Autodesk Inventor part; units mm, degrees
ref_plane "YZ Plane" through (0, 0, 0) normal (1, 0, 0) x (0, 1, 0)
ref_plane "XZ Plane" through (0, 0, 0) normal (0, 1, 0) x (-1, 0, 0)
ref_plane "XY Plane" through (0, 0, 0) normal (0, 0, 1) x (1, 0, 0)
sketch "Esquisse1" plane through (0, 0, 0) normal (0, 1, 0) x (-1, 0, 0)
  line L0 (0, 0) -> (20, 0)
  line L1 (20, 0) -> (20, -86)
  line L2 (20, -86) -> (0, -86)
  line L3 (0, -86) -> (0, 0)
  dimension "d0" = 86
  dimension "d1" = 20
extrude "Extrusion1" add sketch "Esquisse1" along normal blind 3
sketch "Esquisse2" plane through (0, 3, 0) normal (0, 1, 0) x (1, 0, 0)
  line L0 (-20, 0) -> (0, 0)
  line L1 (0, 0) -> (0, 86)
  line L2 (10.8927, 42.5) -> (-28.8955, 42.5) construction
  point P0 (-3, 6)
  dimension "d12" = 3
  dimension "d37" = 42.5
  dimension "d39" = 36.5
hole "Perçage1" at (-3, 3, -6) direction (0, -1, 0) diameter 3.5 end through all
pattern_linear "Réseau rectangulaire1" count 2 spacing 14 along (-1, 0, 0) count 2 spacing 74 along (0, 0, -1) of "Perçage1"
sketch "Esquisse3" plane through (0, 3, 0) normal (0, 1, 0) x (1, 0, 0)
  line L0 (-15.25, 31) -> (-2.75, 31)
  line L1 (-2.75, 31) -> (-2.75, 55)
  line L2 (-2.75, 55) -> (-15.25, 55)
  line L3 (-15.25, 55) -> (-15.25, 31)
  line L4 (0, 86) -> (-20, 86)
  line L5 (-20, 86) -> (-20, 0)
  point P0 (0, 0)
  dimension "d19" = 24
  dimension "d20" = 12.5
  dimension "d21" = 31
  dimension "d22" = 4.75
extrude "Extrusion2" cut sketch "Esquisse3" against normal through all
sketch "Esquisse4" plane through (0, 3, 0) normal (0, 1, 0) x (1, 0, 0)
  line L0 (-2.75, 55) -> (-2.75, 31)
  line L1 (-2.75, 31) -> (-15.25, 31)
  point P0 (0, 0)
  point P1 (-9, 29.15)
  dimension "d32" = 6.25
  dimension "d33" = 1.85
hole "Perçage2" at (-9, 3, -29.15) direction (0, -1, 0) diameter 2 end through all
pattern_linear "Réseau rectangulaire2" count 2 spacing 27.7 along (0, 0, -1) of "Perçage2"
properties part number "support_servo_moteur"
Build history of the part. All positions in model axes, mm. A direction names the side the tool comes from. Round coordinates to 2 decimals unless told otherwise and drop trailing zeros. Write each loop counter-clockwise with the first axis right and the second up, starting at its lowest first coordinate (ties: lowest second). Pieces come first, ordered by that corner, then holes. Notation, with made-up numbers: M 60.25,61.5 L 79.25,61.5 A17 ccw 79.25,78.5 Z; hole C 58,27.25 d8. An arc over 180 degrees is marked long. Answer as a JSON object with one key per item and string values. Group by question number.
(1) Cut at C-C (y = 0.95). Give the cut face in (x, z).
(2) Which spindle directions (+Z, -Z, +X, -X, +Y, -Y) get a long thin tool onto all of the face, cutting with end or side? Do faces 1 (the flat face through (-2.75, 2, -43)), 2 (the flat face through (0, 1, -44)). Say none if no direction does.
(3) Mould opens along X. For faces 3 (the flat face through (-9, 2, -31)), 4 (the flat face through (-10, 1, 0)), 5 (the flat face through (-20, 1, -42)) say: pulls with the +X half, pulls with the -X half, needs draft (parallel to the pull), parting line crosses it, or undercut.
(4) Drill centre lines: L1, parallel to Z at x = -17, y = 0.85; L2, parallel to Z at x = -3, y = 1.3; L3, parallel to Z at x = -9, y = 1.9. Where is each one in solid material? Low to high.
(5) Cut at B-B (x = -9). Give the cut face in (y, z), and give its area (3 significant figures).
(6) Cut at D-D (x = -17). Give the cut face in (y, z).
(7) Cut at A-A (z = -6). Give the cut face in (x, y).
Responses:
{
 "1": {"outline": "M -20,-86 L 0,-86 L 0,0 L -20,0 Z; hole C -17,-80 d3.5; hole C -17,-6 d3.5; hole M -15.25,-55 L -2.75,-55 L -2.75,-31 L -15.25,-31 Z; hole C -9,-56.85 d2; hole C -9,-29.15 d2; hole C -3,-80 d3.5; hole C -3,-6 d3.5"},
 "2": {"face 1": "+Y, -Y", "face 2": "+Z, -Z, +X, +Y, -Y"},
 "3": {"face 3": "undercut", "face 4": "needs draft", "face 5": "pulls with the -X half"},
 "4": {"L1": "z = -86 to -81.75, -78.25 to -7.75, -4.25 to 0", "L2": "z = -86 to -81.75, -78.25 to -55, -31 to -7.75, -4.25 to 0", "L3": "z = -86 to -57.85, -55.85 to -55, -31 to -30.15, -28.15 to 0"},
 "5": {"outline": "M 0,-86 L 3,-86 L 3,-57.85 L 0,-57.85 Z; M 0,-55.85 L 3,-55.85 L 3,-55 L 0,-55 Z; M 0,-31 L 3,-31 L 3,-30.15 L 0,-30.15 Z; M 0,-28.15 L 3,-28.15 L 3,0 L 0,0 Z", "area": "174 mm2"},
 "6": {"outline": "M 0,-86 L 3,-86 L 3,-81.75 L 0,-81.75 Z; M 0,-78.25 L 3,-78.25 L 3,-7.75 L 0,-7.75 Z; M 0,-4.25 L 3,-4.25 L 3,0 L 0,0 Z"},
 "7": {"outline": "M -20,0 L -18.75,0 L -18.75,3 L -20,3 Z; M -15.25,0 L -4.75,0 L -4.75,3 L -15.25,3 Z; M -1.25,0 L 0,0 L 0,3 L -1.25,3 Z"}
}
